Geometry check sheet. Reference: the model listing, model coordinates, mm. Face numbers are marked on the shaded views. A direction names the side the tool comes from. Coordinates: 2 decimals unless noted, no trailing zeros. Loops run counter-clockwise (first coordinate to the right, second up) from the corner with the lowest first, then second, coordinate; pieces in that order, holes last. Notation, with made-up numbers: M -18,16.5 L 3,16.5 A28 cw 3,35.5 Z; hole C 85.25,74.5 d8. An arc over 180 degrees is marked long. Use CSV: the item, a comma, the result in double quotes.
```python
from build123d import *

# Parameters (mm, degrees)
SKETCH1_W           = 58
SKETCH1_H           = 25
SKETCH1_R           = 1.9
BOSS_EXTRUDE1_DEPTH = 3
SKETCH2_R           = 6
BOSS_EXTRUDE2_DEPTH = 20
SKETCH3_R           = 4
CUT_EXTRUDE1_DEPTH  = 38.379807383
SKETCH4_W           = 7.7
SKETCH4_H           = 19.996282454
BOSS_EXTRUDE3_DEPTH = 19
CUT_EXTRUDE2_REACH  = 57.325
SKETCH5_R           = 4
FILLET1_R           = 4
SKETCH7_W           = 4.2
SKETCH7_H           = 25
BOSS_EXTRUDE4_DEPTH = 3
SKETCH8_W           = 5
SKETCH8_H           = 19.996282454
BOSS_EXTRUDE5_DEPTH = 19
CUT_EXTRUDE3_REACH  = 64.547
SKETCH9_R           = 4
FILLET2_R           = 4


with BuildPart() as part:
    # Sketch1 → Boss-Extrude1 (new body)
    with BuildSketch(Plane.XY):
        Rectangle(SKETCH1_W, SKETCH1_H)
        with Locations((24.2, 5)):
            Circle(SKETCH1_R, mode=Mode.SUBTRACT)
        with Locations((24.2, -5)):
            Circle(SKETCH1_R, mode=Mode.SUBTRACT)
        with Locations((-24.2, 5)):
            Circle(SKETCH1_R, mode=Mode.SUBTRACT)
        with Locations((-24.2, -5)):
            Circle(SKETCH1_R, mode=Mode.SUBTRACT)
    extrude(amount=BOSS_EXTRUDE1_DEPTH)

    # Sketch2 → Boss-Extrude2 (add)
    with BuildSketch(Plane.XY):
        Circle(SKETCH2_R)
    extrude(amount=BOSS_EXTRUDE2_DEPTH)

    # Sketch3 → Cut-Extrude1 (cut, through all)
    with BuildSketch(Plane.XY.offset(20)):
        Circle(SKETCH3_R)
    extrude(amount=-CUT_EXTRUDE1_DEPTH, mode=Mode.SUBTRACT)

    # Sketch4 → Boss-Extrude3 (add)
    with BuildSketch(Plane.XY.offset(3)):
        with Locations((-16.35, 0)):
            Rectangle(SKETCH4_W, SKETCH4_H)
    extrude(amount=BOSS_EXTRUDE3_DEPTH)

    # Sketch5 → Cut-Extrude2 (cut, up to next)
    with BuildSketch(Plane.ZY.offset(20.2), mode=Mode.PRIVATE) as cut_extrude2_sk1:
        with Locations((15.5, 0.080826905)):
            Circle(SKETCH5_R)
    cut_extrude2_tool1 = extrude(cut_extrude2_sk1.sketch, amount=-CUT_EXTRUDE2_REACH, mode=Mode.PRIVATE) & part.part
    add(cut_extrude2_tool1.solids().sort_by_distance((-20.2, 0.080827, 15.5))[0], mode=Mode.SUBTRACT)

    # Fillet1
    fillet1_edges = [part.edges().sort_by_distance(p)[0] for p in [
        (-16.35, 9.998141227, 22),
        (-16.35, -9.998141227, 22),
    ]]
    fillet(fillet1_edges, radius=FILLET1_R)

    # Sketch7 → Boss-Extrude4 (add)
    with BuildSketch(Plane.XY.offset(3)):
        with Locations((-31.1, 0)):
            Rectangle(SKETCH7_W, SKETCH7_H)
    extrude(amount=-BOSS_EXTRUDE4_DEPTH)

    # Sketch8 → Boss-Extrude5 (add)
    with BuildSketch(Plane.XY.offset(3)):
        with Locations((-30.7, 0)):
            Rectangle(SKETCH8_W, SKETCH8_H)
    extrude(amount=BOSS_EXTRUDE5_DEPTH)

    # Sketch9 → Cut-Extrude3 (cut, up to next)
    with BuildSketch(Plane(origin=(-28.2, 0, 0), x_dir=(0, 0, -1), z_dir=(1, 0, 0)), mode=Mode.PRIVATE) as cut_extrude3_sk1:
        with Locations(Location((-15.5, 0.063578072, 0), (0, 0, 90))):
            Circle(SKETCH9_R)
    cut_extrude3_tool1 = extrude(cut_extrude3_sk1.sketch, amount=-CUT_EXTRUDE3_REACH, mode=Mode.PRIVATE) & part.part
    add(cut_extrude3_tool1.solids().sort_by_distance((-28.2, 0.063578, 15.5))[0], mode=Mode.SUBTRACT)

    # Fillet2
    fillet2_edges = [part.edges().sort_by_distance(p)[0] for p in [
        (-30.7, 9.998141227, 22),
        (-30.7, -9.998141227, 22),
    ]]
    fillet(fillet2_edges, radius=FILLET2_R)


solid = part.part
```
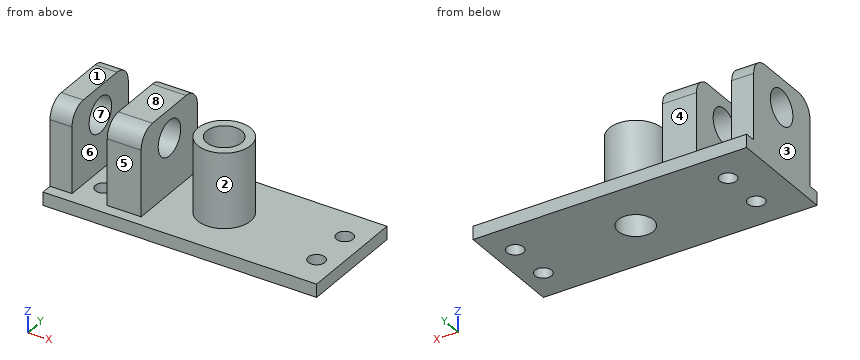
1. Set-up check for the marked faces 4, 5, 6, 7 and 8: record each of +Z, -Z, +X, -X, +Y, -Y from which the full face is reachable in a straight line by a thin tool's end or side.
The answers:
face 4,"+Z, +X, -X, +Y"
face 5,"+Z, +X, -X, -Y"
face 6,"+Z, +Y, -Y"
face 7,"-X"
face 8,"+Z, +X, -X, +Y, -Y"
2. Release check for a two-part mould opening along X. For the marked faces 1, 2 and 3 record: +X half, -X half, draft (parallel to the pull), parting line (faces both ways), or undercut.
The answers:
face 1,"draft"
face 2,"undercut"
face 3,"-X half"
3. Section check A-A, the plane z = 15.5. Record the cut outline in (x, y), plus the area to 3 significant figures.
The answers:
outline,"M -33.2,-10 L -28.2,-10 L -28.2,-3.94 L -33.2,-3.94 Z; M -33.2,4.06 L -28.2,4.06 L -28.2,10 L -33.2,10 Z; M -20.2,-10 L -12.5,-10 L -12.5,-3.92 L -20.2,-3.92 Z; M -20.2,4.08 L -12.5,4.08 L -12.5,10 L -20.2,10 Z; C 0,0 d12; hole C 0,0 d8"
area,"215 mm^2"
4. Section check B-B, the plane x = 0. Record the cut outline in (y, z).
The answers:
outline,"M -12.5,0 L -4,0 L -4,20 L -6,20 L -6,3 L -12.5,3 Z; M 4,0 L 12.5,0 L 12.5,3 L 6,3 L 6,20 L 4,20 Z"
5. Thickness scan on line 1 (Y direction, x = 24.2, z = 1.95); line 2 (X direction, y = 6.5, z = 10.5); line 3 (X direction, y = 2.5, z = 10). Record the ranges inside material, lowest first. Write a range as [from, to].
The answers:
line 1,"[-12.5, -6.9], [-3.1, 3.1], [6.9, 12.5]"
line 2,"[-33.2, -28.2], [-20.2, -12.5]"
line 3,"[-33.2, -28.2], [-20.2, -12.5], [-5.45, -3.12], [3.12, 5.45]"
6. Section check D-D, the plane x = -14. Record the cut outline in (y, z), plus the area to 3 significant figures.
The answers:
outline,"M -12.5,0 L 12.5,0 L 12.5,3 L 10,3 L 10,18 A4 ccw 6,22 L -6,22 A4 ccw -10,18 L -10,3 L -12.5,3 Z; hole C 0.08,15.5 d8"
area,"398 mm^2"
7. Section check C-C, the plane y = -0.75. Record the cut outline in (x, z), plus the area to 3 significant figures.
The answers:
outline,"M -33.2,0 L -3.93,0 L -3.93,20 L -5.95,20 L -5.95,3 L -12.5,3 L -12.5,11.59 L -20.2,11.59 L -20.2,3 L -28.2,3 L -28.2,11.58 L -33.2,11.58 Z; M -33.2,19.42 L -28.2,19.42 L -28.2,22 L -33.2,22 Z; M -20.2,19.41 L -12.5,19.41 L -12.5,22 L -20.2,22 Z; M 3.93,0 L 29,0 L 29,3 L 5.95,3 L 5.95,20 L 3.93,20 Z"
area,"374 mm^2"
8. Gauge pin test, flat ends, axial feed: P1, Ø6, axis at x = -1.5, y = 0, coming from the +Z side; P2, Ø5.5, axis at x = -31, z = 13, coming from the -Y side; P3, Ø6, axis at x = -24.2, y = 5, coming from the +Z side; P4, Ø2.5, axis at x = 24.2, y = 5, coming from the +Z side. Record the tip position at first contact, or that the pin passes through.
The answers:
P1,"z = 20"
P2,"y = -10"
P3,"z = 3"
P4,"through"
